Here's how the part is built. I have some questions about the finished solid (model axes, mm). Round coordinates to 2 decimals unless told otherwise and drop trailing zeros. Loops run counter-clockwise (first coordinate to the right, second up) from the corner with the lowest first, then second, coordinate; pieces in that order, holes last. Notation, with made-up numbers: M 30.5,7 L 49.5,7 A25 cw 49.5,44 Z; hole C 70.5,3.25 d5. An arc over 180 degrees is marked long. Answer as a JSON object with one key per item and string values.
from build123d import *

# Parameters (mm, degrees)
SKETCH1_W           = 152.4
SKETCH1_H           = 53.721
BOSS_EXTRUDE1_DEPTH = 50.8
SKETCH2_R           = 5
CUT_EXTRUDE1_DEPTH  = 19.416667
SKETCH2_4_R         = 5.5
SKETCH2_4_R_2       = 5
CUT_EXTRUDE2_DEPTH  = 5.254167
SKETCH2_5_R         = 7.5
SKETCH2_5_R_2       = 5.5
CUT_EXTRUDE3_DEPTH  = 4.123106


with BuildPart() as part:
    # Sketch1 → Boss-Extrude1 (new body)
    with BuildSketch(Plane(origin=(0, 0, 0), x_dir=(1, 0, 0), z_dir=(0, 1, 0))):
        Rectangle(SKETCH1_W, SKETCH1_H)
    extrude(amount=BOSS_EXTRUDE1_DEPTH)

    # Sketch2 → Cut-Extrude1 (cut)
    with BuildSketch(Plane(origin=(0, 50.8, 0), x_dir=(1, 0, 0), z_dir=(0, 1, 0))):
        with Locations(Location((0, 0, 0), (0, 0, 270))):
            Circle(SKETCH2_R)
    extrude(amount=-CUT_EXTRUDE1_DEPTH, mode=Mode.SUBTRACT)

    # Sketch2_4 → Cut-Extrude2 (cut)
    with BuildSketch(Plane(origin=(0, 50.8, 0), x_dir=(1, 0, 0), z_dir=(0, 1, 0))):
        with Locations(Location((0, 0, 0), (0, 0, 270))):
            Circle(SKETCH2_4_R)
        with Locations(Location((0, 0, 0), (0, 0, 270))):
            Circle(SKETCH2_4_R_2, mode=Mode.SUBTRACT)
    extrude(amount=-CUT_EXTRUDE2_DEPTH, mode=Mode.SUBTRACT)

    # Sketch2_5 → Cut-Extrude3 (cut)
    with BuildSketch(Plane(origin=(0, 50.8, 0), x_dir=(1, 0, 0), z_dir=(0, 1, 0))):
        with Locations(Location((-1, 0, 0), (0, 0, 270))):
            Circle(SKETCH2_5_R)
        with Locations(Location((0, 0, 0), (0, 0, 270))):
            Circle(SKETCH2_5_R_2, mode=Mode.SUBTRACT)
    extrude(amount=-CUT_EXTRUDE3_DEPTH, mode=Mode.SUBTRACT)


solid = part.part
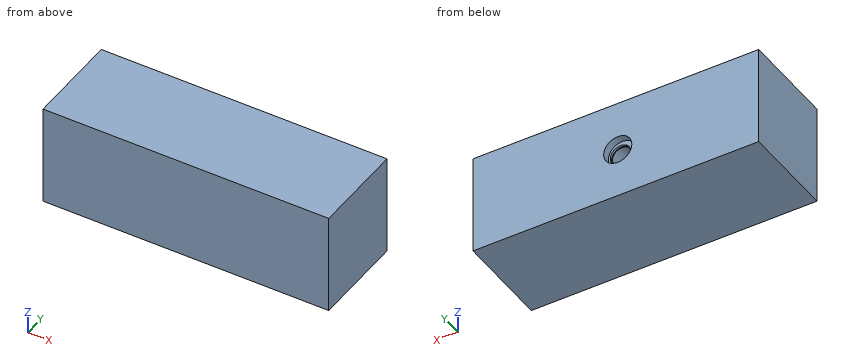
Item 1: For P1, Ø3, axis at x = 2, z = -1, coming from the +Y side; P2, Ø12, axis at x = -1, z = 0, coming from the +Y side, each with a flat end and sliding along its axis, tell me the tip position at first contact or that it passes through.
Solution:
{"P1": "stops at y = 31.38", "P2": "stops at y = 46.68"}
Item 2: If I drill on L1, parallel to X at y = 34, z = 0; L2, parallel to X at y = 49, z = 0, over which ranges is the centre line in solid material (lowest first)? Write a range as from..to.
Solution:
{"L1": "x = -76.2..-5, 5..76.2", "L2": "x = -76.2..-8.5, 6.5..76.2"}
Item 3: I want a section at A-A on z = 0. List the corners of the cut face in (x, y) for me, plus the area to 3 significant figures.
Solution:
{"outline": "M -76.2,0 L 76.2,0 L 76.2,50.8 L 6.5,50.8 L 6.5,46.68 L 5.5,46.68 L 5.5,45.55 L 5,45.55 L 5,31.38 L -5,31.38 L -5,45.55 L -5.5,45.55 L -5.5,46.68 L -8.5,46.68 L -8.5,50.8 L -76.2,50.8 Z", "area": "7,530 mm2"}
